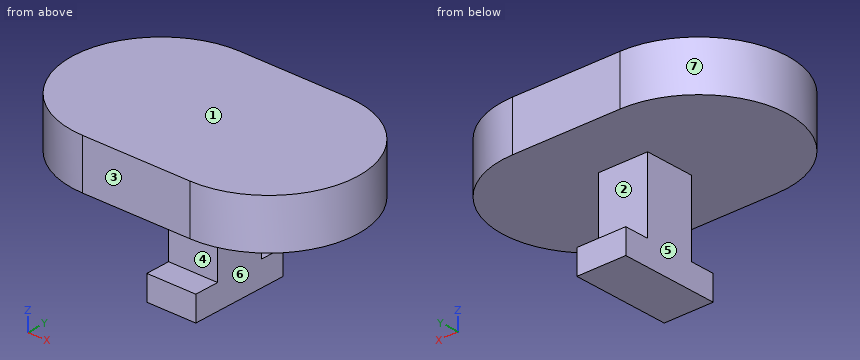
```python
from build123d import *

# Parameters (mm, degrees)
BOSS_EXTRUDE1_DEPTH = 1.27
SKETCH5_W           = 1.27
SKETCH5_H           = 1.27
BOSS_EXTRUDE2_DEPTH = 1.905
SKETCH6_W           = 1.27
SKETCH6_H           = 2.54
BOSS_EXTRUDE3_DEPTH = 0.635


with BuildPart() as part:
    # Sketch3 → Boss-Extrude1 (new body)
    with BuildSketch(Plane.XY):
        with BuildLine():
            Line((-1.397, 2.286), (1.397, 2.286))
            ThreePointArc((1.397, 2.286), (3.683, 0), (1.397, -2.286))
            Line((1.397, -2.286), (-1.397, -2.286))
            ThreePointArc((-1.397, -2.286), (-3.683, 0), (-1.397, 2.286))
        make_face()
    extrude(amount=-BOSS_EXTRUDE1_DEPTH)

    # Sketch5 → Boss-Extrude2 (add)
    with BuildSketch(Plane(origin=(0, 0, -1.27), x_dir=(-1, 0, 0), z_dir=(0, 0, -1))):
        Rectangle(SKETCH5_W, SKETCH5_H)
    extrude(amount=BOSS_EXTRUDE2_DEPTH)

    # Sketch6 → Boss-Extrude3 (add)
    with BuildSketch(Plane(origin=(0, 0, -3.175), x_dir=(-1, 0, 0), z_dir=(0, 0, -1))):
        Rectangle(SKETCH6_W, SKETCH6_H)
    extrude(amount=BOSS_EXTRUDE3_DEPTH)


solid = part.part
```
Design review of the part built by this model. Coordinates are the model's own, in mm. Face numbers are marked on the shaded views. A direction names the side the tool comes from. Give positions to 0.01 mm unless a question says otherwise; leave off trailing zeros. Write each loop counter-clockwise with the first axis right and the second up, starting at its lowest first coordinate (ties: lowest second). Pieces come first, ordered by that corner, then holes.
(1) Add section D-D (z = -0.35). Give the boundary of the cut face in (x, y), and give its area (3 significant figures).
Checked values:
outline: (-1.4, -2.29) - (1.4, -2.29) arc R2.29 ccw to (1.4, 2.29) - (-1.4, 2.29) arc R2.29 ccw to start
area: 29.2 mm2
(2) Tool access review of the marked faces 4, 5, 6 and 7: name each direction out of +Z, -Z, +X, -X, +Y, -Y from which nothing blocks a thin tool from reaching the whole face with its end or side.
Checked values:
face 4: +X, -X, -Y
face 5: -Z, -X, +Y, -Y
face 6: -Z, +X, +Y, -Y
face 7: +Z, -Z, -X
(3) Mouldability with a two-part tool opening along Z and no side actions: class the marked faces 1, 2 and 3 as +Z half, -Z half, draft (parallel to the pull), parting line (faces both ways), or undercut.
Checked values:
face 1: +Z half
face 2: undercut
face 3: draft
(4) Wall thickness on line 1 along Z through (x, y) = (-0.25, -0.95) (3 decimals); line 2 along X through (y, z) = (0.4, -2.7) (3 decimals); line 3 along Z through (x, y) = (3, 1): over which ranges is each line inside the solid? List them lowest first.
Checked values:
line 1: z = -3.81 to -3.175, -1.27 to 0
line 2: x = -0.635 to 0.635
line 3: z = -1.27 to 0
(5) Add section C-C (x = 0.5). Give the boundary of the cut face in (y, z) (3 decimals).
Checked values:
outline: (-2.286, -1.27) - (-0.635, -1.27) - (-0.635, -3.175) - (-1.27, -3.175) - (-1.27, -3.81) - (1.27, -3.81) - (1.27, -3.175) - (0.635, -3.175) - (0.635, -1.27) - (2.286, -1.27) - (2.286, 0) - (-2.286, 0) - close
(6) Add section A-A (y = 0). Give the boundary of the cut face in (x, z) (3 decimals).
Checked values:
outline: (-3.683, -1.27) - (-0.635, -1.27) - (-0.635, -3.81) - (0.635, -3.81) - (0.635, -1.27) - (3.683, -1.27) - (3.683, 0) - (-3.683, 0) - close
(7) Add section B-B (y = -1.15). Give the boundary of the cut face in (x, z) (3 decimals), and give its area (3 significant figures).
Checked values:
outline: (-3.373, -1.27) - (3.373, -1.27) - (3.373, 0) - (-3.373, 0) - close; (-0.635, -3.81) - (0.635, -3.81) - (0.635, -3.175) - (-0.635, -3.175) - close
area: 9.37 mm2
(8) Clearance check with flat-ended pins moving along their axes: pin 1 Ø0.7 at (x, z) = (0.5, -3.5) entering from +Y; pin 2 Ø2 at (y, z) = (-0.5, -3) entering from +X (3 decimals); pin 3 Ø0.5 at (x, z) = (0, -3.5) entering from -Y. State where each tip first meets the part, or that it passes through.
Checked values:
pin 1: stops at y = 1.27
pin 2: stops at x = 0.635
pin 3: stops at y = -1.27
